Geometry check sheet. Reference: the model listing, model coordinates, mm. A direction names the side the tool comes from. Round coordinates to 2 decimals unless told otherwise and drop trailing zeros. Write each loop counter-clockwise with the first axis right and the second up, starting at its lowest first coordinate (ties: lowest second). Pieces come first, ordered by that corner, then holes. Notation, with made-up numbers: M 59,-35.5 L 72,-35.5 A25 ccw 72,-13.5 Z; hole C 6.25,16.25 d3. An arc over 180 degrees is marked long. Use a Markdown table: item, result.
```python
from build123d import *

# Parameters (mm, degrees)
SKETCH1_W           = 33.9
SKETCH1_H           = 30
BOSS_EXTRUDE5_DEPTH = 3
SKETCH3_R           = 2.5
CUT_EXTRUDE2_DEPTH  = 3
SKETCH7_W           = 33.9
SKETCH7_H           = 30
BOSS_EXTRUDE6_DEPTH = 3
SKETCH8_R           = 3.8
CUT_EXTRUDE3_DEPTH  = 3
SKETCH10_R          = 3.8
CUT_EXTRUDE4_DEPTH  = 3


with BuildPart() as part:
    # Sketch1 → Boss-Extrude5 (new body)
    with BuildSketch(Plane.XY):
        Rectangle(SKETCH1_W, SKETCH1_H)
    extrude(amount=BOSS_EXTRUDE5_DEPTH)

    # Sketch3 → Cut-Extrude2 (cut)
    with BuildSketch(Plane.XY.offset(3)):
        with Locations((-11.95, 9)):
            Circle(SKETCH3_R)
        with Locations((11.95, 9)):
            Circle(SKETCH3_R)
        with Locations((11.95, -9)):
            Circle(SKETCH3_R)
        with Locations((-11.95, -9)):
            Circle(SKETCH3_R)
    extrude(amount=-CUT_EXTRUDE2_DEPTH, mode=Mode.SUBTRACT)

    # Sketch7 → Boss-Extrude6 (add)
    with BuildSketch(Plane.XY.offset(3)):
        Rectangle(SKETCH7_W, SKETCH7_H)
    extrude(amount=BOSS_EXTRUDE6_DEPTH)

    # Sketch8 → Cut-Extrude3 (cut)
    with BuildSketch(Plane(origin=(0, 0, 3), x_dir=(-1, 0, 0), z_dir=(0, 0, -1))):
        with Locations((11.95, 9)):
            Circle(SKETCH8_R)
    extrude(amount=-CUT_EXTRUDE3_DEPTH, mode=Mode.SUBTRACT)

    # Sketch10 → Cut-Extrude4 (cut)
    with BuildSketch(Plane(origin=(0, 0, 3), x_dir=(-1, 0, 0), z_dir=(0, 0, -1))):
        with Locations((-11.95, 9)):
            Circle(SKETCH10_R)
        with Locations((-11.95, -9)):
            Circle(SKETCH10_R)
        with Locations((11.95, -9)):
            Circle(SKETCH10_R)
    extrude(amount=-CUT_EXTRUDE4_DEPTH, mode=Mode.SUBTRACT)


solid = part.part
```
Item 1: Cross-section at B-B, the plane x = 11.95. Record the cut outline in (y, z), and give its area (3 significant figures).
Outcome:
| item | result |
|---|---|
| outline | M -15,0 L -11.5,0 L -11.5,3 L -12.8,3 L -12.8,6 L -15,6 Z; M -6.5,0 L 6.5,0 L 6.5,3 L 5.2,3 L 5.2,6 L -5.2,6 L -5.2,3 L -6.5,3 Z; M 11.5,0 L 15,0 L 15,6 L 12.8,6 L 12.8,3 L 11.5,3 Z |
| area | 104 mm2 |
Item 2: Access from +Z, -Z, +X, -X, +Y, -Y to the whole of each face (thin tool, end or side, straight path). Record for faces 4 (the face through (0, 0, 0)), 5 (the face through (-12, -6, 3)).
Outcome:
| item | result |
|---|---|
| face 4 | -Z, +X, -X, +Y, -Y |
| face 5 | +Z |
Item 3: Go/stop test with a flat-tipped pin: pin 1 (6 mm diameter, centred on x = 11.95, y = -9, fed in from +Z). Record where the tip stops, or that it passes through.
Outcome:
| item | result |
|---|---|
| pin 1 | stops at z = 3 |
Item 4: Mould release check, pull along X, two halves, no side actions. Record for faces 1 (the face through (-16.95, 0, 3)), 2 (the face through (0, 15, 3)), 3 (the face through (9.9, -5.8, 4.5)): +X half, -X half, draft (parallel to the pull), parting line (faces both ways), or undercut.
Outcome:
| item | result |
|---|---|
| face 1 | -X half |
| face 2 | draft |
| face 3 | undercut |
Item 5: Material ranges on line 1 along Y through (x, z) = (-11.95, 4.6); line 2 along Y through (x, z) = (-11.95, 2.3); line 3 along X through (y, z) = (7.75, 4.55), recorded low to high. Write a range as from..to.
Outcome:
| item | result |
|---|---|
| line 1 | y = -15..-12.8, -5.2..5.2, 12.8..15 |
| line 2 | y = -15..-11.5, -6.5..6.5, 11.5..15 |
| line 3 | x = -16.95..-15.54, -8.36..8.36, 15.54..16.95 |
Item 6: Cross-section at D-D, the plane z = 4.4. Record the cut outline in (x, y).
Outcome:
| item | result |
|---|---|
| outline | M -16.95,-15 L 16.95,-15 L 16.95,15 L -16.95,15 Z; hole C -11.95,-9 d7.6; hole C -11.95,9 d7.6; hole C 11.95,-9 d7.6; hole C 11.95,9 d7.6 |
Item 7: Cross-section at C-C, the plane y = 9. Record the cut outline in (x, z).
Outcome:
| item | result |
|---|---|
| outline | M -16.95,0 L -14.45,0 L -14.45,3 L -15.75,3 L -15.75,6 L -16.95,6 Z; M -9.45,0 L 9.45,0 L 9.45,3 L 8.15,3 L 8.15,6 L -8.15,6 L -8.15,3 L -9.45,3 Z; M 14.45,0 L 16.95,0 L 16.95,6 L 15.75,6 L 15.75,3 L 14.45,3 Z |
Item 8: Cross-section at A-A, the plane z = 1.65. Record the cut outline in (x, y).
Outcome:
| item | result |
|---|---|
| outline | M -16.95,-15 L 16.95,-15 L 16.95,15 L -16.95,15 Z; hole C -11.95,-9 d5; hole C -11.95,9 d5; hole C 11.95,-9 d5; hole C 11.95,9 d5 |
